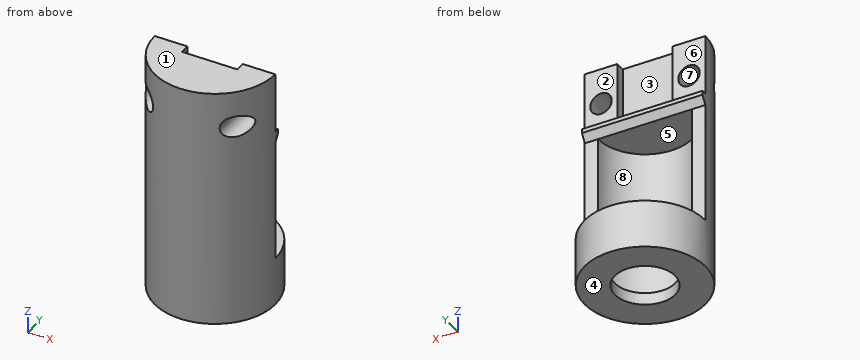
from build123d import *

# Parameters (mm, degrees)
SKETCH1_R               = 6.35
BOSS_EXTRUDE1_DEPTH     = 12.7
SKETCH3_W               = 12.7
SKETCH3_H               = 15.24
CUT_EXTRUDE2_DEPTH      = 7.35
CUT_EXTRUDE3_START      = -2.54
SKETCH4_R               = 4.953
CUT_EXTRUDE3_DEPTH      = 6.35
CUT_EXTRUDE3_DEPTH_BACK = 6.35
SKETCH5_R               = 3.175
CUT_EXTRUDE4_DEPTH      = 2.27
SKETCH7_W               = 5.842
SKETCH7_H               = 6.35
CUT_EXTRUDE5_DEPTH      = 1.016
SKETCH8_R               = 1.1303
CUT_EXTRUDE6_DEPTH      = 7.35
SKETCH10_R              = 4.953
CUT_EXTRUDE7_DEPTH      = 16.51
SKETCH11_W              = 12.869582419
SKETCH11_H              = 6.56213844
CUT_EXTRUDE8_DEPTH      = 12.7
BOSS_EXTRUDE2_DEPTH     = 6.35


with BuildPart() as part:
    # Sketch1 → Boss-Extrude1 (new body, symmetric)
    with BuildSketch(Plane.XY):
        Circle(SKETCH1_R)
    extrude(amount=BOSS_EXTRUDE1_DEPTH, both=True)

    # Sketch3 → Cut-Extrude2 (cut, through all)
    with BuildSketch(Plane(origin=(0, 0, 0), x_dir=(1, 0, 0), z_dir=(0, 1, 0))):
        with Locations((0, -5.08)):
            Rectangle(SKETCH3_W, SKETCH3_H)
    extrude(amount=CUT_EXTRUDE2_DEPTH, mode=Mode.SUBTRACT)

    # Sketch4 → Cut-Extrude3 (cut, two sides)
    with BuildSketch(Plane.XY.offset(-2.54).offset(CUT_EXTRUDE3_START)) as cut_extrude3_sk:
        Circle(SKETCH4_R)
    extrude(amount=CUT_EXTRUDE3_DEPTH, mode=Mode.SUBTRACT)
    extrude(cut_extrude3_sk.sketch, amount=-CUT_EXTRUDE3_DEPTH_BACK, mode=Mode.SUBTRACT)

    # Sketch5 → Cut-Extrude4 (cut, through all)
    with BuildSketch(Plane.XY.offset(-11.43)):
        Circle(SKETCH5_R)
    extrude(amount=-CUT_EXTRUDE4_DEPTH, mode=Mode.SUBTRACT)

    # Sketch7 → Cut-Extrude5 (cut)
    with BuildSketch(Plane(origin=(0, 0, 0), x_dir=(1, 0, 0), z_dir=(0, 1, 0))):
        with Locations((0, -9.525)):
            Rectangle(SKETCH7_W, SKETCH7_H)
    extrude(amount=-CUT_EXTRUDE5_DEPTH, mode=Mode.SUBTRACT)

    # Sketch8 → Cut-Extrude6 (cut, through all)
    with BuildSketch(Plane(origin=(0, 0, 0), x_dir=(1, 0, 0), z_dir=(0, 1, 0))):
        with Locations((-4.6355, -8.89)):
            Circle(SKETCH8_R)
        with Locations((4.6355, -8.89)):
            Circle(SKETCH8_R)
    extrude(amount=-CUT_EXTRUDE6_DEPTH, mode=Mode.SUBTRACT)

    # Sketch10 → Cut-Extrude7 (cut)
    with BuildSketch(Plane.XY.offset(-11.43)):
        Circle(SKETCH10_R)
    extrude(amount=CUT_EXTRUDE7_DEPTH, mode=Mode.SUBTRACT)

    # Sketch11 → Cut-Extrude8 (cut)
    with BuildSketch(Plane(origin=(0, 0, 5.08), x_dir=(-1, 0, 0), z_dir=(0, 0, -1))):
        with Locations((-0.08479121, 3.28106922)):
            Rectangle(SKETCH11_W, SKETCH11_H)
    extrude(amount=CUT_EXTRUDE8_DEPTH, mode=Mode.SUBTRACT)

    # Sketch12 → Boss-Extrude2 (add, symmetric)
    with BuildSketch(Plane(origin=(0, 0, 0), x_dir=(0, 0, -1), z_dir=(1, 0, 0))):
        Polygon((-6.35, 0), (-5.08, 0), (-5.9270724, 0.508), (-6.35, 0.508), align=None)
    extrude(amount=BOSS_EXTRUDE2_DEPTH, both=True)


solid = part.part
Could you check a few things on this model? Use its own coordinates, in mm. Face numbers are marked on the shaded views. A direction names the side the tool comes from. Round coordinates to 2 decimals unless told otherwise and drop trailing zeros. Write each loop counter-clockwise with the first axis right and the second up, starting at its lowest first coordinate (ties: lowest second). Pieces come first, ordered by that corner, then holes. Notation, with made-up numbers: (75, 51) - (96, 51) arc R24 cw to (96, 74) - close; hole circle Ø7 at (58, -32). An arc over 180 degrees is marked (long way). Use a Markdown table: item, result.
Q1. Please list where these lines run through material, in increasing order: L1, parallel to Z at x = -3, y = -2; L2, parallel to Y at x = 0, z = -11.85 (3 decimals); L3, parallel to X at y = -1.45, z = 8.89.
Output values:
| item | result |
|---|---|
| L1 | -12.7 to -11.43, 5.08 to 12.7 |
| L2 | -6.35 to -3.175, 3.175 to 6.35 |
| L3 | -6.18 to -5.77, -3.51 to 3.51, 5.77 to 6.18 |
Q2. Thinking about a two-plate mould opening in Y: for the marked faces 6, 7 and 8, which applies, released by +Y, released by -Y, zero draft, split by the parting line, or undercut?
Output values:
| item | result |
|---|---|
| face 6 | released by +Y |
| face 7 | zero draft |
| face 8 | undercut |
Q3. I want a section at A-A (x = 0). List the corners of the cut face in (y, z) for me (3 decimals), plus the area to 3 significant figures.
Output values:
| item | result |
|---|---|
| outline | (-6.35, -12.7) - (-3.175, -12.7) - (-3.175, -11.43) - (-4.953, -11.43) - (-4.953, 5.08) - (0, 5.08) - (0.508, 5.927) - (0.508, 6.35) - (-1.016, 6.35) - (-1.016, 12.7) - (-6.35, 12.7) - close; (3.175, -12.7) - (6.35, -12.7) - (6.35, -7.62) - (4.953, -7.62) - (4.953, -11.43) - (3.175, -11.43) - close |
| area | 78.8 mm2 |
Q4. For the marked faces 1, 2, 3, 4 and 5, which set-ups out of +Z, -Z, +X, -X, +Y, -Y let a thin tool reach every point of the face, with its end or its side?
Output values:
| item | result |
|---|---|
| face 1 | +Z, +X, -X, +Y, -Y |
| face 2 | +Z, +X, -X, +Y |
| face 3 | +Z, +Y |
| face 4 | -Z, +X, -X, +Y, -Y |
| face 5 | +Y |
Q5. I want a section at B-B (z = 8.89). List the corners of the cut face in (x, y) for me.
Output values:
| item | result |
|---|---|
| outline | (-6.35, 0) arc R6.35 ccw to (-5.77, -2.66) - (-5.77, 0) - close; (-3.51, -5.29) arc R6.35 ccw to (3.51, -5.29) - (3.51, 0) - (2.92, 0) - (2.92, -1.02) - (-2.92, -1.02) - (-2.92, 0) - (-3.51, 0) - close; (5.77, -2.66) arc R6.35 ccw to (6.35, 0) - (5.77, 0) - close |
Q6. For pin 1 (1.1 mm diameter, centred on x = 6, z = 1.5, fed in from +Y); pin 2 (1 mm diameter, centred on y = -4, z = -1, fed in from +X); pin 3 (5 mm diameter, centred on x = -0.5, y = 2, fed in from +Z); pin 4 (2 mm diameter, centred on y = 3, z = 6.5, fed in from +X), each with a flat end and sliding along its axis, tell me the tip position at first contact or that it passes through.
Output values:
| item | result |
|---|---|
| pin 1 | y = 0 |
| pin 2 | x = 5.3 |
| pin 3 | z = 6.35 |
| pin 4 | through |
Q7. I want a section at C-C (y = 1). List the corners of the cut face in (x, z) for me.
Output values:
| item | result |
|---|---|
| outline | (-6.27, -12.7) - (-3.01, -12.7) - (-3.01, -11.43) - (-4.85, -11.43) - (-4.85, -7.62) - (-6.27, -7.62) - close; (3.01, -12.7) - (6.27, -12.7) - (6.27, -7.62) - (4.85, -7.62) - (4.85, -11.43) - (3.01, -11.43) - close |
Q8. I want a section at D-D (y = 4.25). List the corners of the cut face in (x, z) for me.
Output values:
| item | result |
|---|---|
| outline | (-4.72, -12.7) - (4.72, -12.7) - (4.72, -7.62) - (2.54, -7.62) - (2.54, -11.43) - (-2.54, -11.43) - (-2.54, -7.62) - (-4.72, -7.62) - close |
